```python
from build123d import *

# Parameters (mm, degrees)
EXTRUDE_2_DEPTH          = 13
CUT_EXTRUDE_1_DEPTH      = 35.406576406
CUT_EXTRUDE_1_DEPTH_BACK = 35.406576406


with BuildPart() as part:
    # 草图1 → 凸台-拉伸2 (new body)
    with BuildSketch(Plane(origin=(0, 0, 0), x_dir=(1, 0, 0), z_dir=(0, 1, 0))):
        with BuildLine():
            Line((0.75, 15), (2.5, 0))
            ThreePointArc((2.5, 0), (4, -1.5), (5.5, 0))
            Line((5.5, 0), (7.25, 15))
            ThreePointArc((7.25, 15), (8, 15.75), (8.75, 15))
            Line((8.75, 15), (10.5, 0))
            ThreePointArc((10.5, 0), (12, -1.5), (13.5, 0))
            Line((13.5, 0), (15.25, 15))
            ThreePointArc((15.25, 15), (16, 15.75), (16.75, 15))
            Line((16.75, 15), (18.5, 0))
            ThreePointArc((18.5, 0), (20, -1.5), (21.5, 0))
            Line((21.5, 0), (23.25, 15))
            ThreePointArc((23.25, 15), (24, 15.75), (24.75, 15))
            Line((24.75, 15), (26.5, 0))
            Line((26.5, 0), (27.25, 0))
            Line((27.25, 0), (25.5, 15))
            ThreePointArc((25.5, 15), (24, 16.5), (22.5, 15))
            Line((22.5, 15), (20.75, 0))
            ThreePointArc((20.75, 0), (20, -0.75), (19.25, 0))
            Line((19.25, 0), (17.5, 15))
            ThreePointArc((17.5, 15), (16, 16.5), (14.5, 15))
            Line((14.5, 15), (12.75, 0))
            ThreePointArc((12.75, 0), (12, -0.75), (11.25, 0))
            Line((11.25, 0), (9.5, 15))
            ThreePointArc((9.5, 15), (8, 16.5), (6.5, 15))
            Line((6.5, 15), (4.75, 0))
            ThreePointArc((4.75, 0), (4, -0.75), (3.25, 0))
            Line((3.25, 0), (1.5, 15))
            ThreePointArc((1.5, 15), (0, 16.5), (-1.5, 15))
            Line((-1.5, 15), (-3.425, -1.5))
            Line((-3.425, -1.5), (-2.675, -1.5))
            Line((-2.675, -1.5), (-0.75, 15))
            ThreePointArc((-0.75, 15), (0, 15.75), (0.75, 15))
        make_face()
    extrude(amount=EXTRUDE_2_DEPTH)

    # 草图2 → 切除-拉伸1 (cut, two sides: drawn at the far end of the back side and taken through both)
    with BuildSketch(Plane(origin=(0, 0, 0), x_dir=(0, 0, -1), z_dir=(1, 0, 0)).offset(-CUT_EXTRUDE_1_DEPTH_BACK)):
        with BuildLine():
            Line((7.5, 13), (-1.5, 13))
            Line((-1.5, 13), (-1.5, 9.38083152))
            ThreePointArc((-1.5, 9.38083152), (2.649784013, 12.061318538), (7.5, 13))
        make_face()
        with BuildLine():
            Line((16.5, 13), (7.5, 13))
            ThreePointArc((7.5, 13), (12.350215987, 12.061318538), (16.5, 9.38083152))
            Line((16.5, 9.38083152), (16.5, 13))
        make_face()
    extrude(amount=CUT_EXTRUDE_1_DEPTH + CUT_EXTRUDE_1_DEPTH_BACK, mode=Mode.SUBTRACT)


solid = part.part
```
CAD build for the part. Positions are in the model's coordinates, mm. A direction names the side the tool comes from. Give positions to 0.01 mm unless a question says otherwise; leave off trailing zeros. Loops run counter-clockwise (first coordinate to the right, second up) from the corner with the lowest first, then second, coordinate; pieces in that order, holes last. Notation, with made-up numbers: (52, 56) -> (106, 56) arc R22 ccw to (106, 76) -> close; hole circle Ø3 at (32, 23). An arc over 180 degrees is marked (long way). Use a Markdown table: item, result.
1. Slice it at D-D (x = 10). List the corners of the cut face in (y, z).
Check result:
| item | result |
|---|---|
| outline | (0, -10.71) -> (12.6, -10.71) arc R13 ccw to (12.6, -4.29) -> (0, -4.29) -> close |
2. Slice it at A-A (z = -14.5). Give the number of separate pieces and of enclosed holes in the cut face, plus the area to 3 significant figures.
Check result:
| item | result |
|---|---|
| separate pieces | 8 |
| enclosed holes | 0 |
| area | 65.7 mm^2 |
3. Which spindle directions (+Z, -Z, +X, -X, +Y, -Y) get a long thin tool onto all of the face, cutting with end or side? Do faces 1 (the flat face through (14.363, 6.409, -7.395)), 2 (the flat face through (21.637, 6.409, -7.605)). Say none if no direction does.
Check result:
| item | result |
|---|---|
| face 1 | +Z, +Y, -Y |
| face 2 | -Z, +Y, -Y |
4. Wall check: L1, parallel to Z at x = 16, y = 6; L2, parallel to Y at x = 14.5, z = -13.5; L3, parallel to Y at x = 6, z = -4.75. Give the ranges that are in metal, low to high. Write a range as [from, to].
Check result:
| item | result |
|---|---|
| L1 | z = [-16.5, -15.75] |
| L2 | y = [0, 11.53] |
| L3 | y = [0, 12.71] |
5. Flat gauge pins, fed straight in: pin 1 (4 mm diameter, centred on x = 21.5, z = -9.5, fed in from +Y); pin 2 (2 mm diameter, centred on x = 3, z = -5.5, fed in from +Y); pin 3 (4 mm diameter, centred on y = 6, z = -3.5, fed in from -X) (3 decimals). Where does each tip first touch, or does it go through?
Check result:
| item | result |
|---|---|
| pin 1 | stops at y = 13 |
| pin 2 | stops at y = 12.95 |
| pin 3 | stops at x = -3.075 |
6. Mould opens along X. For faces 3 (the flat face through (13.637, 6.409, -7.605)), 4 (the flat face through (-2.45, 6.41, -6.87)) say: pulls with the +X half, pulls with the -X half, needs draft (parallel to the pull), parting line crosses it, or undercut.
Check result:
| item | result |
|---|---|
| face 3 | undercut |
| face 4 | pulls with the -X half |
